Could you check a few things on this model? Use its own coordinates, in mm. Face numbers are marked on the shaded views. Coordinates: 2 decimals unless noted, no trailing zeros. Loops run counter-clockwise (first coordinate to the right, second up) from the corner with the lowest first, then second, coordinate; pieces in that order, holes last. Notation, with made-up numbers: (37.5, 23.5) -> (69.5, 23.5) arc R17 cw to (69.5, 37.5) -> close; hole circle Ø5 at (26, -10). An arc over 180 degrees is marked (long way). One line per question, with ' | ' between items.
```python
from build123d import *

# Parameters (mm, degrees)
F2_R      = 15.875
F3_DEPTH  = 1.778
F4_W      = 0.889
F4_H      = 1.778
F6_R      = 5.08
F12_DEPTH = 25.4


# Not quite as in the source:
# - a fillet or chamfer that OpenCascade refuses, or shapes differently, is made with other operations: its cross-section is extruded or revolved along the edge and cut away or added


with BuildPart() as f1:
    # F0 (on Front) → F1 (revolve)
    with BuildSketch(Plane.XZ):
        Polygon((8.89, 16.51), (0, 16.51), (0, 3.302), (10.9728, 3.302), align=None)
        Polygon((10.9728, 3.302), (0, 3.302), (0, 1.27), (11.2932307692, 1.27), (10.9728, 1.8250023726), align=None)
        Polygon((11.2932307692, 1.27), (0, 1.27), (0, -4.318), (12.1744153846, -4.318), align=None)
        Polygon((12.1744153846, -4.318), (0, -4.318), (0, -6.35), (12.4948461538, -6.35), (12.1744153846, -5.7949976274), align=None)
        Polygon((12.4948461538, -6.35), (0, -6.35), (0, -16.51), (14.097, -16.51), align=None)
    revolve(axis=Axis((0, 0, 0), (0, 0, -1)))

    # F2 (on face) → F3 (join)
    with BuildSketch(Plane(origin=(0, 0, -16.51), x_dir=(1, 0, 0), z_dir=(0, 0, -1))):
        Circle(F2_R)
    extrude(amount=-F3_DEPTH)

    # F4 (on Front) → F5 (revolve, cut)
    with BuildSketch(Plane.XZ):
        with Locations((13.4747296192, -13.843)):
            Rectangle(F4_W, F4_H)
    revolve(axis=Axis((0, 0, -8.2004386932), (0, 0, -1)), mode=Mode.SUBTRACT)

    # F6
    f6_edges = [f1.edges().sort_by_distance(p)[0] for p in [
        (-12.174415, 0, -4.318),
        (-10.9728, 0, 3.302),
    ]]
    fillet(f6_edges, radius=F6_R)

    # F7: fillet of radius 5.08 on 2 edges, made by hand

    # F7_s1 → F7_t2 (revolve, cut)
    with BuildSketch(Plane.XZ):
        with BuildLine():
            ThreePointArc((10.9728, 1.8250023726), (11.259283136, 1.1139138917), (11.4354988153, 0.367812391))
            Line((11.4354988153, 0.367812391), (11.2932307692, 1.27))
            Line((11.2932307692, 1.27), (10.9728, 1.8250023726))
        make_face()
    revolve(axis=Axis((0, 0, 1.27), (0, 0, -1)), mode=Mode.SUBTRACT)

    # F7_s3 → F7_t4 (revolve, cut)
    with BuildSketch(Plane.XZ):
        with BuildLine():
            ThreePointArc((12.1744153846, -5.7949976274), (12.4608985206, -6.5060861083), (12.6371141999, -7.252187609))
            Line((12.6371141999, -7.252187609), (12.4948461538, -6.35))
            Line((12.4948461538, -6.35), (12.1744153846, -5.7949976274))
        make_face()
    revolve(axis=Axis((0, 0, -6.35), (0, 0, -1)), mode=Mode.SUBTRACT)

    # F11 (on line) → F12 (cut)
    with BuildSketch(Plane(origin=(0, 8.524875, 8.524875), x_dir=(-1, 0, 0), z_dir=(0, 0.7071067812, 0.7071067812))):
        with BuildLine():
            Line((8.8735996043, 11.2926720722), (0.53975, 11.2926720722))
            Line((0.53975, 11.2926720722), (0.53975, 5.3997505037))
            Line((0.53975, 5.3997505037), (7.62, -2.9089047656))
            add(Edge.make_bspline(
                [(8.8735996043, 11.2926720722), (8.9393181622, 8.7279276849), (9.2979393658, 4.1523383564), (7.9516483041, -0.3346072044), (7.62, -2.9089047656)],
                knots=[0, 0, 0, 0, 0.4980817697, 1, 1, 1, 1], degree=3))
        make_face()
        with BuildLine():
            Line((-0.53975, 5.3997505037), (-0.53975, 11.2926720722))
            Line((-0.53975, 11.2926720722), (-8.8735996043, 11.2926720722))
            add(Edge.make_bspline(
                [(-8.8735996043, 11.2926720722), (-8.9393181622, 8.7279276849), (-9.2979393658, 4.1523383564), (-7.9516483041, -0.3346072044), (-7.62, -2.9089047656)],
                knots=[0, 0, 0, 0, 0.4980817697, 1, 1, 1, 1], degree=3))
            Line((-7.62, -2.9089047656), (-0.53975, 5.3997505037))
        make_face()
    extrude(amount=F12_DEPTH, mode=Mode.SUBTRACT)


solid = f1.part
```
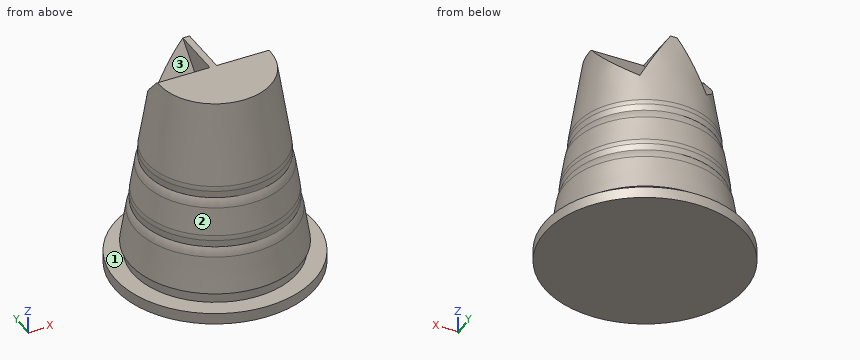
Q1. For pin 1 (4.5 mm diameter, centred on y = 3.5, z = 15, fed in from -X); pin 2 (6 mm diameter, centred on x = -10, z = 6, fed in from +Y); pin 3 (5 mm diameter, centred on x = 1, z = 13, fed in from +Y), each with a flat end and sliding along its axis, tell me the tip position at first contact or that it passes through.
Values follow:
pin 1: stops at x = -9.19 | pin 2: stops at y = 7.96 | pin 3: stops at y = 9.82
Q2. Please list where these lines run through material, in increasing order: L1, parallel to Y at x = 9, z = -7.5; L2, parallel to Z at x = -7, y = -12.5; L3, parallel to X at y = -9.5, z = -8. Write a range as [from, to].
Values follow:
L1: y = [-8.93, 8.93] | L2: z = [-16.51, -14.73] | L3: x = [-8.51, 8.51]
Q3. Imagine slicing it at A-A on z = 9. Write out the boundary of the cut face in (x, y), plus the area to 3 significant figures.
Values follow:
outline: (-6.06, 8.05) arc R10.07 ccw (long way) to (6.06, 8.05) -> (4.57, 8.05) -> (4.99, 8.75) arc R10.07 ccw to (-4.99, 8.75) -> (-4.57, 8.05) -> close | area: 318 mm2
Q4. Imagine slicing it at B-B on z = -2. Write out the boundary of the cut face in (x, y).
Values follow:
outline: circle Ø23.62 at (0, 0)
Q5. We'd pull the mould along Y, two halves only. Please class the marked faces 1, 2 and 3: released by +Y, released by -Y, zero draft, split by the parting line, or undercut.
Values follow:
face 1: zero draft | face 2: split by the parting line | face 3: undercut
